Verification items for the finished model (mm, model axes). Give positions to 0.01 mm unless a question says otherwise; leave off trailing zeros. Order: outer loops, then holes, each group sorted by start corner. A loop starts at its lowest first (then second) coordinate and runs counter-clockwise, first axis right, second up.
(1) Scan lines: L1, parallel to Z at x = 0, y = -133; L2, parallel to Z at x = 187, y = -189.5; L3, parallel to X at y = -158, z = -109.5. Record each from-to range of solid material in increasing order.
(2) Sectioned sample at C-C on y = -150. Record the cut outline in (x, z), plus the area to 3 significant figures.
(3) Sectioned sample at A-A on z = 0. Record the cut outline in (x, y), plus the area to 3 significant figures.
(4) Sectioned sample at B-B on x = -18.5. Record the cut outline in (y, z).
(5) Gauge pin test, flat ends, axial feed: pin 1 (2 mm diameter, centred on x = 47.5, y = -154, fed in from +Z); pin 2 (1.1 mm diameter, centred on y = -73, z = -228.5, fed in from -X); pin 3 (1.1 mm diameter, centred on y = -102.5, z = -103, fed in from +X). Record the tip position at first contact, or that the pin passes through.
(6) Sectioned sample at D-D on z = -113.5. Record the cut outline in (x, y), plus the area to 3 significant figures.
Autodesk Inventor part; units mm, degrees
ref_plane "YZ Plane" through (0, 0, 0) normal (1, 0, 0) x (0, 1, 0)
ref_plane "XZ Plane" through (0, 0, 0) normal (0, 1, 0) x (-1, 0, 0)
ref_plane "XY Plane" through (0, 0, 0) normal (0, 0, 1) x (1, 0, 0)
sketch "Sketch1" plane through (0, 0, 0) normal (0, 1, 0) x (-1, 0, 0)
  circle A0 centre (0, 0) radius 228.6
  circle A1 centre (0, 0) radius 227.5764
  line L0 (0, 0) -> (0, 228.6) construction
  line L1 (0, 0) -> (-228.6, 0) construction
  line L2 (0, 0) -> (228.6, 0) construction
  line L3 (0, 0) -> (0, -228.6) construction
  dimension "d0" = 1.0236
  dimension "d1" = 457.2
ref_plane "Work Plane1" through (0, 0, 228.6) normal (0, 0, 1) x (1, 0, 0)
ref_plane "Work Plane2" through (-228.6, 0, 0) normal (-1, 0, 0) x (0, -1, 0)
ref_plane "Work Plane3" through (0, 0, -228.6) normal (0, 0, -1) x (-1, 0, 0)
ref_plane "Work Plane4" through (228.6, 0, 0) normal (1, 0, 0) x (0, 1, 0)
extrude "Extrusion1" add sketch "Sketch1" against normal blind 203.2
sketch "Sketch2" plane through (0, 0, -228.6) normal (0, 0, -1) x (-1, 0, 0)
  line L0 (-228.6, -203.2) -> (228.6, -203.2) construction
  line L1 (0, 0) -> (0, -50.8) construction
  line L2 (0, -127) -> (0, -50.8) construction
  line L3 (0, -127) -> (25.4, -127)
  line L4 (25.4, -127) -> (25.4, -50.8)
  line L5 (25.4, -50.8) -> (0, -50.8)
  line L6 (0, -127) -> (0, -50.8)
  line L7 (-228.6, 0) -> (-228.6, -203.2)
  point P0 (228.6, 0)
  dimension "d4" = 50.8
  dimension "d9" = 76.2
  dimension "d10" = 25.4
extrude "Extrusion2" cut sketch "Sketch2" against normal blind 228.6
sketch "Sketch3" plane through (0, 0, -228.6) normal (0, 0, -1) x (-1, 0, 0)
  line L0 (0, -127) -> (25.4, -127)
  line L1 (203.2, -50.8) -> (0, -50.8)
  line L2 (0, -50.8) -> (0, -127)
  line L3 (0, -127) -> (203.2, -127)
  line L4 (203.2, -127) -> (203.2, -50.8)
  point P0 (0, 0)
  point P1 (203.2, -133.35)
extrude "Extrusion3" cut sketch "Sketch3" against normal blind 228.6
properties part number "Cyclone Main Straight Metal"
Ans:
1. L1: z = -228.6 to -227.58, 227.58 to 228.6
1. L2: z = -131.49 to -129.7, 129.7 to 131.49
1. L3: x = -200.67 to -199.5, 199.5 to 200.67
2. outline: circle Ø457.2 at (0, 0); hole circle Ø455.15 at (0, 0)
2. area: 1,470 mm2
3. outline: (-228.6, -203.2) - (-227.58, -203.2) - (-227.58, 0) - (-228.6, 0) - close; (227.58, -203.2) - (228.6, -203.2) - (228.6, 0) - (227.58, 0) - close
3. area: 416 mm2
4. outline: (-203.2, -227.85) - (-127, -227.85) - (-127, -226.82) - (-203.2, -226.82) - close; (-203.2, 226.82) - (0, 226.82) - (0, 227.85) - (-203.2, 227.85) - close; (-50.8, -227.85) - (0, -227.85) - (0, -226.82) - (-50.8, -226.82) - close
5. pin 1: stops at z = 223.82
5. pin 2: stops at x = 0
5. pin 3: stops at x = 204.36
6. outline: (-198.43, -203.2) - (-197.25, -203.2) - (-197.25, -127) - (-198.43, -127) - close; (-198.43, -50.8) - (-197.25, -50.8) - (-197.25, 0) - (-198.43, 0) - close; (197.25, -203.2) - (198.43, -203.2) - (198.43, 0) - (197.25, 0) - close
6. area: 390 mm2
